```python
from build123d import *

# Parameters (mm, degrees)
F0_R     = 19.05
F1_DEPTH = 38.1
F2_DEPTH = 25.4
F3_DEPTH = 31.75


with BuildPart() as f1:
    # F0 (on Top) → F1 (new body)
    with BuildSketch(Plane.XY):
        with BuildLine():
            ThreePointArc((-37.6632987603, -10.0267366713), (-22.1449503188, -1.4965177663), (-15.972041403, 15.1010413445))
            ThreePointArc((-15.972041403, 15.1010413445), (-21.7134087863, 31.1851379508), (-36.3419755478, 39.9979977347))
            Line((-36.3419755478, 39.9979977347), (-41.3982813704, 40.5010277907))
            ThreePointArc((-41.3982813704, 40.5010277907), (-66.762647964, 14.4103181957), (-40.0173078877, -10.2628049155))
            Line((-40.0173078877, -10.2628049155), (-37.6632987603, -10.0267366713))
        make_face()
        with Locations((-41.372041403, 15.1010413445)):
            Circle(F0_R, mode=Mode.SUBTRACT)
    extrude(amount=F1_DEPTH)

    # F0 (on Top) → F2 (join)
    with BuildSketch(Plane.XY):
        with BuildLine():
            ThreePointArc((-36.3419755478, 39.9979977347), (-21.7134087863, 31.1851379508), (-15.972041403, 15.1010413445))
            Line((-15.972041403, 15.1010413445), (-9.622041403, 15.1010413445))
            ThreePointArc((-9.622041403, 15.1010413445), (-7.7621694636, 19.5911694051), (-3.272041403, 21.4510413445))
            Line((-3.272041403, 21.4510413445), (47.527958597, 21.4510413445))
            ThreePointArc((47.527958597, 21.4510413445), (52.0180866575, 19.5911694051), (53.877958597, 15.1010413445))
            Line((53.877958597, 15.1010413445), (72.927958597, 15.1010413445))
            ThreePointArc((72.927958597, 15.1010413445), (77.1037936501, 24.5153183725), (86.8852203227, 27.7386555558))
            Line((86.8852203227, 27.7386555558), (-36.3419755478, 39.9979977347))
        make_face()
        with BuildLine():
            Line((-9.622041403, 15.1010413445), (-15.972041403, 15.1010413445))
            ThreePointArc((-15.972041403, 15.1010413445), (-22.1449503188, -1.4965177663), (-37.6632987603, -10.0267366713))
            Line((-37.6632987603, -10.0267366713), (86.8952026298, 2.4644242117))
            ThreePointArc((86.8952026298, 2.4644242117), (77.1075125763, 5.6833983481), (72.927958597, 15.1010413445))
            Line((72.927958597, 15.1010413445), (53.877958597, 15.1010413445))
            ThreePointArc((53.877958597, 15.1010413445), (52.0180866575, 10.610913284), (47.527958597, 8.7510413445))
            Line((47.527958597, 8.7510413445), (-3.272041403, 8.7510413445))
            ThreePointArc((-3.272041403, 8.7510413445), (-7.7621694636, 10.610913284), (-9.622041403, 15.1010413445))
        make_face()
    extrude(amount=F2_DEPTH)

    # F0 (on Top) → F3 (join)
    with BuildSketch(Plane.XY):
        with BuildLine():
            ThreePointArc((98.327958597, 15.1010413445), (95.0422356249, 23.6252062914), (86.8852203227, 27.7386555558))
            ThreePointArc((86.8852203227, 27.7386555558), (77.1037936501, 24.5153183725), (72.927958597, 15.1010413445))
            ThreePointArc((72.927958597, 15.1010413445), (77.1075125763, 5.6833983481), (86.8952026298, 2.4644242117))
            ThreePointArc((86.8952026298, 2.4644242117), (95.0456015934, 6.5805953238), (98.327958597, 15.1010413445))
        make_face()
        with BuildLine():
            ThreePointArc((91.977958597, 15.1010413445), (85.627958597, 8.7510413445), (79.277958597, 15.1010413445))
            ThreePointArc((79.277958597, 15.1010413445), (85.627958597, 21.4510413445), (91.977958597, 15.1010413445))
        make_face(mode=Mode.SUBTRACT)
    extrude(amount=F3_DEPTH)


solid = f1.part
```
Geometry check sheet. Reference: the model listing, model coordinates, mm. A direction names the side the tool comes from. Coordinates: 2 decimals unless noted, no trailing zeros. Loops run counter-clockwise (first coordinate to the right, second up) from the corner with the lowest first, then second, coordinate; pieces in that order, holes last. Notation, with made-up numbers: (-10, -2) -> (45, -2) arc R22 ccw to (45, 31) -> close; hole circle Ø8 at (27.5, 21.5). An arc over 180 degrees is marked (long way). Put each result on its own line as item: value.
1) Tool access check on faces 1 (the flat face through (79.8, 18.1, 31.75)), 2 (the flat face through (-37.7, 34, 38.1)), 3 (the flat face through (22, 21.451, 13)). Record the directions out of +Z, -Z, +X, -X, +Y, -Y that give a thin tool (end or side, any length) a straight path to the whole face; none if there is none.
Result set:
face 1: +Z, +X, +Y, -Y
face 2: +Z, +X, -X, +Y, -Y
face 3: +Z, -Z
2) Gauge pin test, flat ends, axial feed: pin 1 Ø1.5 at (x, z) = (66, 6) entering from +Y; pin 2 Ø8 at (x, y) = (47.5, 32.5) entering from -Z; pin 3 Ø10 at (x, z) = (6.5, 21.5) entering from +Y; pin 4 Ø7.5 at (x, z) = (25, 18.5) entering from +Y. Record the tip position at first contact, or that the pin passes through.
Result set:
pin 1: stops at y = 29.89
pin 2: stops at z = 0
pin 3: stops at y = 36.23
pin 4: stops at y = 34.27
3) Release check for a two-part mould opening along X. For faces 4 (the cylindrical face through (-55.41, 27.98, 18.78)), 5 (the flat face through (15, 27, 0)) record: released by +X, released by -X, zero draft, split by the parting line, or undercut.
Result set:
face 4: undercut
face 5: zero draft
4) Thickness scan on line 1 (X direction, y = 15, z = 34); line 2 (X direction, y = 10.5, z = 22.5); line 3 (X direction, y = 20.5, z = 17). Record the ranges inside material, lowest first.
Result set:
line 1: x = -66.77 to -60.42, -22.32 to -15.97
line 2: x = -66.35 to -59.86, -22.89 to -7.65, 51.9 to 81.25, 90 to 97.47
line 3: x = -66.19 to -59.64, -23.1 to -6.61, 50.87 to 82.29, 88.97 to 97.12
5) Cross-section at C-C on z = 18.5. Record the boundary of the cut face in (x, y).
Result set:
outline: (-41.4, 40.5) arc R25.4 ccw (long way) to (-40.02, -10.26) -> (86.9, 2.46) arc R12.7 ccw to (86.89, 27.74) -> close; hole circle Ø38.1 at (-41.37, 15.1); hole (-3.27, 8.75) -> (47.53, 8.75) arc R6.35 ccw to (47.53, 21.45) -> (-3.27, 21.45) arc R6.35 ccw to start; hole circle Ø12.7 at (85.63, 15.1)
6) Cross-section at B-B on x = -56. Record the boundary of the cut face in (y, z), plus the area to 3 significant figures.
Result set:
outline: (-5.66, 0) -> (2.9, 0) -> (2.9, 38.1) -> (-5.66, 38.1) -> close; (27.3, 0) -> (35.87, 0) -> (35.87, 38.1) -> (27.3, 38.1) -> close
area: 652 mm^2
7) Cross-section at D-D on y = 0.5. Record the boundary of the cut face in (x, z), plus the area to 3 significant figures.
Result set:
outline: (-62.16, 0) -> (-53.61, 0) -> (-53.61, 38.1) -> (-62.16, 38.1) -> close; (-29.14, 0) -> (67.31, 0) -> (67.31, 25.4) -> (-20.59, 25.4) -> (-20.59, 38.1) -> (-29.14, 38.1) -> close
area: 2,880 mm^2
8) Cross-section at A-A on z = 30. Record the boundary of the cut face in (x, y), plus the area to 3 significant figures.
Result set:
outline: (-41.4, 40.5) arc R25.4 ccw (long way) to (-40.02, -10.26) -> (-37.66, -10.03) arc R25.4 ccw to (-36.34, 40) -> close; circle Ø25.4 at (85.63, 15.1); hole circle Ø38.1 at (-41.37, 15.1); hole circle Ø12.7 at (85.63, 15.1)
area: 1,270 mm^2
